Work out the finished part from the listing and answer in its coordinate system (mm). A direction names the side the tool comes from. Give positions to 0.01 mm unless a question says otherwise; leave off trailing zeros. Loops run counter-clockwise (first coordinate to the right, second up) from the corner with the lowest first, then second, coordinate; pieces in that order, holes last.
from build123d import *

# Parameters (mm, degrees)
SKETCH1_W           = 40
SKETCH1_H           = 60
SKETCH1_R           = 1.25
BASE_FLANGE1_DEPTH  = 2.5
SKETCH15_R          = 1
CUT_EXTRUDE3_DEPTH  = 10
JOG3_START          = -2.5
JOG3_OUTLINE_W      = 40
JOG3_OUTLINE_H      = 58.294687966
JOG3_OUTLINE_R      = 1
JOG3_OUTLINE_R_2    = 1.25
JOG3_DEPTH          = 2.5
JOG3_2_OUTLINE_W    = 40
JOG3_2_OUTLINE_H    = 1.705312034
JOG3_2_DEPTH        = 0.332528284
JOG3_START_2        = 19.2634
JOG3_3_OUTLINE_W    = 40
JOG3_3_OUTLINE_H    = 40
JOG3_3_OUTLINE_R    = 1
JOG3_3_OUTLINE_R_2  = 1.25
JOG3_3_DEPTH        = 3.2366
JOG3_4_OUTLINE_W    = 40
JOG3_4_OUTLINE_H    = 20.794687966
JOG3_4_OUTLINE_R    = 1.25
JOG3_4_DEPTH        = 3.2366
JOG3_5_OUTLINE_W    = 40
JOG3_5_OUTLINE_H    = 2.5
JOG3_5_DEPTH        = 20
JOG3_START_3        = 20
JOG3_6_OUTLINE_R    = 1.25
JOG3_6_OUTLINE_R_2  = 1
JOG3_6_DEPTH        = 2.5
JOG3_START_4        = -20
JOG3_7_DEPTH        = 40
JOG4_START          = -20
JOG4_DEPTH          = 40
JOG4_2_DEPTH        = 40
JOG4_START_2        = -3
JOG4_3_OUTLINE_R    = 1.25
JOG4_3_DEPTH        = 4
FILLET1_R           = 10
SKETCH18_R          = 2.5
BOSS_EXTRUDE1_DEPTH = 2.5
SKETCH19_R          = 1
SKETCH19_W          = 23.5
SKETCH19_H          = 12.5
CUT_EXTRUDE4_DEPTH  = 2.5
SKETCH20_R          = 2.5
CUT_EXTRUDE6_DEPTH  = 10
SKETCH23_R          = 2.5
CUT_EXTRUDE7_DEPTH  = 51.062460986
SKETCH24_R          = 5
CUT_EXTRUDE8_DEPTH  = 1.25
SKETCH26_R          = 2.5
CUT_EXTRUDE12_DEPTH = 51.062460987
SKETCH27_W          = 20
SKETCH27_H          = 13.5268
CUT_EXTRUDE13_DEPTH = 61.042487703


with BuildPart() as part:
    # Base-Flange1: sheet metal written as solids
    # Sketch1 → Base-Flange1 (new body)
    with BuildSketch(Plane.XY):
        Rectangle(SKETCH1_W, SKETCH1_H)
        with Locations((10, 15)):
            Circle(SKETCH1_R, mode=Mode.SUBTRACT)
        with Locations(Location((10, -15, 0), (0, 0, 180))):
            Circle(SKETCH1_R, mode=Mode.SUBTRACT)
        with Locations((-10, -15)):
            Circle(SKETCH1_R, mode=Mode.SUBTRACT)
        with Locations(Location((-10, 15, 0), (0, 0, 180))):
            Circle(SKETCH1_R, mode=Mode.SUBTRACT)
    extrude(amount=-BASE_FLANGE1_DEPTH)

    # Sketch15 → Cut-Extrude3 (cut)
    with BuildSketch(Plane.XY):
        with Locations((12, 0)):
            Circle(SKETCH15_R)
        with Locations(Location((-17, 0, 0), (0, 0, 180))):
            Circle(SKETCH15_R)
    extrude(amount=-CUT_EXTRUDE3_DEPTH, mode=Mode.SUBTRACT)

    # Jog3: read off the stored shape, not the designer's step
    # Jog3 outline → Jog3 (cut)
    with BuildSketch(Plane.XY.offset(JOG3_START)):
        with Locations((0, -0.852656017)):
            Rectangle(JOG3_OUTLINE_W, JOG3_OUTLINE_H)
        with Locations((-17, 0)):
            Circle(JOG3_OUTLINE_R, mode=Mode.SUBTRACT)
        with Locations((12, 0)):
            Circle(JOG3_OUTLINE_R, mode=Mode.SUBTRACT)
        with Locations((-10, 15)):
            Circle(JOG3_OUTLINE_R_2, mode=Mode.SUBTRACT)
        with Locations((10, 15)):
            Circle(JOG3_OUTLINE_R_2, mode=Mode.SUBTRACT)
        with Locations((10, -15)):
            Circle(JOG3_OUTLINE_R_2, mode=Mode.SUBTRACT)
        with Locations((-10, -15)):
            Circle(JOG3_OUTLINE_R_2, mode=Mode.SUBTRACT)
    extrude(amount=JOG3_DEPTH, mode=Mode.SUBTRACT)

    # Jog3 2 outline → Jog3 2 (cut)
    with BuildSketch(Plane.XY.offset(JOG3_START)):
        with Locations((0, 29.147343983)):
            Rectangle(JOG3_2_OUTLINE_W, JOG3_2_OUTLINE_H)
    extrude(amount=JOG3_2_DEPTH, mode=Mode.SUBTRACT)

    # Jog3 4 outline → Jog3 4 (add)
    with BuildSketch(Plane.XY.offset(JOG3_START)):
        with Locations((0, 40.397343983)):
            Rectangle(JOG3_4_OUTLINE_W, JOG3_4_OUTLINE_H)
        with Locations((10, 35.794687966)):
            Circle(JOG3_4_OUTLINE_R, mode=Mode.SUBTRACT)
        with Locations((-10, 35.794687966)):
            Circle(JOG3_4_OUTLINE_R, mode=Mode.SUBTRACT)
    extrude(amount=JOG3_4_DEPTH)



with BuildPart() as body_2:
    # Jog3 3 outline → Jog3 3 (new body)
    with BuildSketch(Plane.XY.offset(JOG3_START_2)):
        with Locations((0, 10.794687966)):
            Rectangle(JOG3_3_OUTLINE_W, JOG3_3_OUTLINE_H)
        with Locations((12, 20.794687966)):
            Circle(JOG3_3_OUTLINE_R, mode=Mode.SUBTRACT)
        with Locations((-17, 0)):
            Circle(JOG3_3_OUTLINE_R, mode=Mode.SUBTRACT)
        with Locations((-10, 5.794687966)):
            Circle(JOG3_3_OUTLINE_R_2, mode=Mode.SUBTRACT)
        with Locations((12, 0)):
            Circle(JOG3_3_OUTLINE_R, mode=Mode.SUBTRACT)
        with Locations((10, 5.794687966)):
            Circle(JOG3_3_OUTLINE_R_2, mode=Mode.SUBTRACT)
        with Locations((-17, 20.794687966)):
            Circle(JOG3_3_OUTLINE_R, mode=Mode.SUBTRACT)
        with Locations((-10, 15)):
            Circle(JOG3_3_OUTLINE_R_2, mode=Mode.SUBTRACT)
        with Locations((10, 15)):
            Circle(JOG3_3_OUTLINE_R_2, mode=Mode.SUBTRACT)
    extrude(amount=JOG3_3_DEPTH)


with BuildPart() as part_1:
    add(part.part)

    add(body_2.part)  # Jog3 5 merges body 2
    # Jog3 5 outline → Jog3 5 (add)
    with BuildSketch(Plane.XY):
        with Locations((0, 29.544687966)):
            Rectangle(JOG3_5_OUTLINE_W, JOG3_5_OUTLINE_H)
    extrude(amount=JOG3_5_DEPTH)

    # Jog3 6 outline → Jog3 6 (add)
    with BuildSketch(Plane.XY.offset(JOG3_START_3)):
        with Locations((10, 15)):
            Circle(JOG3_6_OUTLINE_R)
        with Locations((-10, 15)):
            Circle(JOG3_6_OUTLINE_R)
        with Locations((12, 0)):
            Circle(JOG3_6_OUTLINE_R_2)
        with Locations((-17, 0)):
            Circle(JOG3_6_OUTLINE_R_2)
    extrude(amount=JOG3_6_DEPTH)

    # Jog3 7 outline → Jog3 7 (cut)
    with BuildSketch(Plane.YZ.offset(JOG3_START_4)):
        with BuildLine():
            ThreePointArc((28.294687966, 19.2634), (28.078942821, 19.784254855), (27.558087966, 20))
            Line((27.558087966, 20), (-9.205312034, 20))
            Line((-9.205312034, 20), (-9.205312034, 19.2634))
            Line((-9.205312034, 19.2634), (28.294687966, 19.2634))
        make_face()
        with BuildLine():
            ThreePointArc((31.531287966, -2.5), (29.242666158, -1.552021808), (28.294687966, 0.7366))
            Line((28.294687966, 0.7366), (28.294687966, -2.167471716))
            Line((28.294687966, -2.167471716), (30, -2.167471716))
            Line((30, -2.167471716), (30, -2.5))
            Line((30, -2.5), (31.531287966, -2.5))
        make_face()
        with BuildLine():
            Line((31.531287966, 0), (50.794687966, 0))
            Line((50.794687966, 0), (50.794687966, 0.7366))
            Line((50.794687966, 0.7366), (30.794687966, 0.7366))
            ThreePointArc((30.794687966, 0.7366), (31.010433111, 0.215745145), (31.531287966, 0))
        make_face()
        with BuildLine():
            Line((30.794687966, 22.5), (27.558087966, 22.5))
            ThreePointArc((27.558087966, 22.5), (29.846709774, 21.552021808), (30.794687966, 19.2634))
            Line((30.794687966, 19.2634), (30.794687966, 22.5))
        make_face()
    extrude(amount=JOG3_7_DEPTH, mode=Mode.SUBTRACT)

    # Jog4: read off the stored shape, not the designer's step
    # Jog4 outline → Jog4 (cut)
    with BuildSketch(Plane.YZ.offset(JOG4_START)):
        with BuildLine():
            Line((-9.205312034, 20), (10.87962174, 20))
            ThreePointArc((10.87962174, 20), (12.019882984, 21.799110859), (14.031287966, 22.5))
            Line((14.031287966, 22.5), (-9.205312034, 22.5))
            Line((-9.205312034, 22.5), (-9.205312034, 20))
        make_face()
    extrude(amount=JOG4_DEPTH, mode=Mode.SUBTRACT)

    # Jog4 2 outline → Jog4 2 (add)
    with BuildSketch(Plane.YZ.offset(JOG4_START)):
        with BuildLine():
            Line((-9.205312034, 0), (-9.205312034, -2.5))
            Line((-9.205312034, -2.5), (10.058087966, -2.5))
            ThreePointArc((10.058087966, -2.5), (12.346709774, -1.552021808), (13.294687966, 0.7366))
            Line((13.294687966, 0.7366), (13.294687966, 19.2634))
            ThreePointArc((13.294687966, 19.2634), (13.510433111, 19.784254855), (14.031287966, 20))
            Line((14.031287966, 20), (10.87962174, 20))
            ThreePointArc((10.87962174, 20), (10.81599152, 19.634140241), (10.794687966, 19.2634))
            Line((10.794687966, 19.2634), (10.794687966, 0.7366))
            ThreePointArc((10.794687966, 0.7366), (10.578942821, 0.215745145), (10.058087966, 0))
            Line((10.058087966, 0), (-9.205312034, 0))
        make_face()
    extrude(amount=JOG4_2_DEPTH)

    # Jog4 3 outline → Jog4 3 (cut)
    with BuildSketch(Plane.XY.offset(JOG4_START_2)):
        with Locations((-10, 5.794687966)):
            Circle(JOG4_3_OUTLINE_R)
        with Locations((10, 5.794687966)):
            Circle(JOG4_3_OUTLINE_R)
    extrude(amount=JOG4_3_DEPTH, mode=Mode.SUBTRACT)

    # Fillet1
    fillet1_edges = [part_1.edges().sort_by_distance(p)[0] for p in [
        (20, -9.205312034, -1.25),
        (-20, -9.205312034, -1.25),
        (-20, 50.794687966, -1.25),
        (20, 50.794687966, -1.25),
    ]]
    fillet(fillet1_edges, radius=FILLET1_R)

    # Sketch18 → Boss-Extrude1 (add)
    with BuildSketch(Plane.XY.offset(22.5)):
        with Locations((12, 20.794687966)):
            Circle(SKETCH18_R)
        with Locations((-17, 20.794687966)):
            Circle(SKETCH18_R)
    extrude(amount=-BOSS_EXTRUDE1_DEPTH)

    # Sketch19 → Cut-Extrude4 (cut)
    with BuildSketch(Plane(origin=(0, 30.794687966, 0), x_dir=(1, 0, 0), z_dir=(0, 1, 0))):
        with Locations(Location((13.9, -7.5, 0), (0, 0, 270))):
            Circle(SKETCH19_R)
        with Locations(Location((-13.9, -7.5, 0), (0, 0, 90))):
            Circle(SKETCH19_R)
        with Locations((0, -7.5)):
            Rectangle(SKETCH19_W, SKETCH19_H)
    extrude(amount=-CUT_EXTRUDE4_DEPTH, mode=Mode.SUBTRACT)

    # Sketch20 → Cut-Extrude6 (cut)
    with BuildSketch(Plane.XY):
        with Locations((0, 40.794687966)):
            Circle(SKETCH20_R)
        with Locations(Location((0, 0.794687966, 0), (0, 0, 180))):
            Circle(SKETCH20_R)
        with Locations((15, 0.794687966)):
            Circle(SKETCH20_R)
        with Locations(Location((-15, 0.794687966, 0), (0, 0, 180))):
            Circle(SKETCH20_R)
        with Locations(Location((15, 40.794687966, 0), (0, 0, 180))):
            Circle(SKETCH20_R)
        with Locations((-15, 40.794687966)):
            Circle(SKETCH20_R)
    extrude(amount=-CUT_EXTRUDE6_DEPTH, mode=Mode.SUBTRACT)

    # Sketch23 → Cut-Extrude7 (cut, through all)
    with BuildSketch(Plane(origin=(0, 30.794687966, 0), x_dir=(1, 0, 0), z_dir=(0, 1, 0))):
        with Locations(Location((-5.55, -7.5, 0), (0, 0, 270))):
            Circle(SKETCH23_R)
    extrude(amount=-CUT_EXTRUDE7_DEPTH, mode=Mode.SUBTRACT)

    # Sketch24 → Cut-Extrude8 (cut)
    with BuildSketch(Plane(origin=(0, 13.294687966, 0), x_dir=(1, 0, 0), z_dir=(0, 1, 0))):
        with Locations(Location((-5.55, -7.5, 0), (0, 0, 270))):
            Circle(SKETCH24_R)
    extrude(amount=-CUT_EXTRUDE8_DEPTH, mode=Mode.SUBTRACT)

    # Sketch26 → Cut-Extrude12 (cut, through all)
    with BuildSketch(Plane.XZ.offset(-10.794687966)):
        with Locations(Location((9.45, 17.5, 0), (0, 0, 135.141364755))):
            Circle(SKETCH26_R)
    extrude(amount=-CUT_EXTRUDE12_DEPTH, mode=Mode.SUBTRACT)

    # Sketch27 → Cut-Extrude13 (cut, through all)
    with BuildSketch(Plane.XY.offset(22.5)):
        Polygon((20, 50.794687966), (0, 50.794687966), (0, 45.794687966), (-5, 45.794687966), (-5, 35.794687966), (0, 35.794687966), (0, 27.558087966), (20, 27.558087966), align=None)
        with Locations((10, 20.794687966)):
            Rectangle(SKETCH27_W, SKETCH27_H)
        Polygon((20, -9.205312034), (20, 14.031287966), (0, 14.031287966), (0, 5.794687966), (5, 5.794687966), (5, -4.205312034), (0, -4.205312034), (0, -9.205312034), align=None)
    extrude(amount=-CUT_EXTRUDE13_DEPTH, mode=Mode.SUBTRACT)


solid = part_1.part
Item 1: Find section B-B, the plane x = -13.9. Give the number of separate pieces and of enclosed holes in the cut face, plus the area to 3 significant figures.
Item 2: Flat-ended cylindrical pins translate along their axes: pin 1 Ø0.8 at (y, z) = (49.5, -1.5) entering from +X; pin 2 Ø6 at (x, y) = (-6, 46) entering from +Z; pin 3 Ø5 at (x, z) = (-7, 18) entering from -Y. Find the tip coordinate at first contact, or state that the pin passes through.
Item 3: Consider line 1 (X direction, y = 29.65, z = 7.5); line 2 (Y direction, x = -10, z = -1.55); line 3 (Y direction, x = -17.5, z = 19). Determine where each line is inside the solid, lowest interval first.
Item 4: Determine the mould class of faces 1 (the face through (0, 32, -1)), 2 (the face through (2.5, 0.7, -1.2)), 3 (the face through (-12, 30.795, 12)) for opening direction Y: released by +Y, released by -Y, zero draft, split by the parting line, or undercut.
Item 5: For faces 4 (the face through (0, -7, -1)), 5 (the face through (2, 5.795, -1)), 6 (the face through (-10, 10.795, 10)), determine the directions among +Z, -Z, +X, -X, +Y, -Y from which every point of the face is accessible in a straight line to the end or side of a thin tool.
Item 6: Find section C-C, the plane y = 29.5. Write down the section's boundary in (x, z), plus the area to 3 significant figures.
Item 7: Find section A-A, the plane z = 7.5. Write down the section's boundary in (x, y), plus the area to 3 significant figures.
Ans:
1. separate pieces: 4
1. enclosed holes: 0
1. area: 223 mm2
2. pin 1: stops at x = 0
2. pin 2: stops at z = 0
2. pin 3: stops at y = 10.79
3. line 1: x = -20 to -14.9, -12.9 to -11.75
3. line 2: y = -9.21 to 4.54, 7.04 to 12.35, 29.24 to 34.54, 37.04 to 50.79
3. line 3: y = 10.79 to 13.29, 28.29 to 30.79
4. face 1: zero draft
4. face 2: undercut
4. face 3: released by +Y
5. face 4: +Z, -Z, +X, -Y
5. face 5: +Z, -Z, +X, +Y
5. face 6: +Z, +X, -X, -Y
6. outline: (-20, -1.78) - (0, -1.78) - (0, 1.25) - (-11.75, 1.25) - (-11.75, 13.75) - (0, 13.75) - (0, 21.85) - (-20, 21.85) - close; hole circle Ø2 at (-13.9, 7.5)
6. area: 323 mm2
7. outline: (-20, 10.79) - (-8.05, 10.79) - (-8.05, 12.04) - (-10.55, 12.04) - (-10.55, 13.29) - (-20, 13.29) - close; (-20, 28.29) - (-14.9, 28.29) - (-14.9, 30.79) - (-20, 30.79) - close; (-12.9, 28.29) - (-11.75, 28.29) - (-11.75, 30.79) - (-12.9, 30.79) - close; (-3.05, 10.79) - (0, 10.79) - (0, 13.29) - (-0.55, 13.29) - (-0.55, 12.04) - (-3.05, 12.04) - close
7. area: 46.9 mm2
